Geometry: see drawing. Coordinates: mm, zero at the bounding-box minimum. A direction names the side the tool comes from. Give positions to 0.01 mm unless a question says otherwise; leave off trailing zeros. Loops run counter-clockwise (first coordinate to the right, second up) from the corner with the lowest first, then second, coordinate; pieces in that order, holes last. Notation, with made-up numbers: M 84,-10 L 139,-10 A32 cw 139,16 Z; hole C 66,-21.5 d10. An arc over 180 degrees is marked long. Answer in a Markdown table with one row per item.
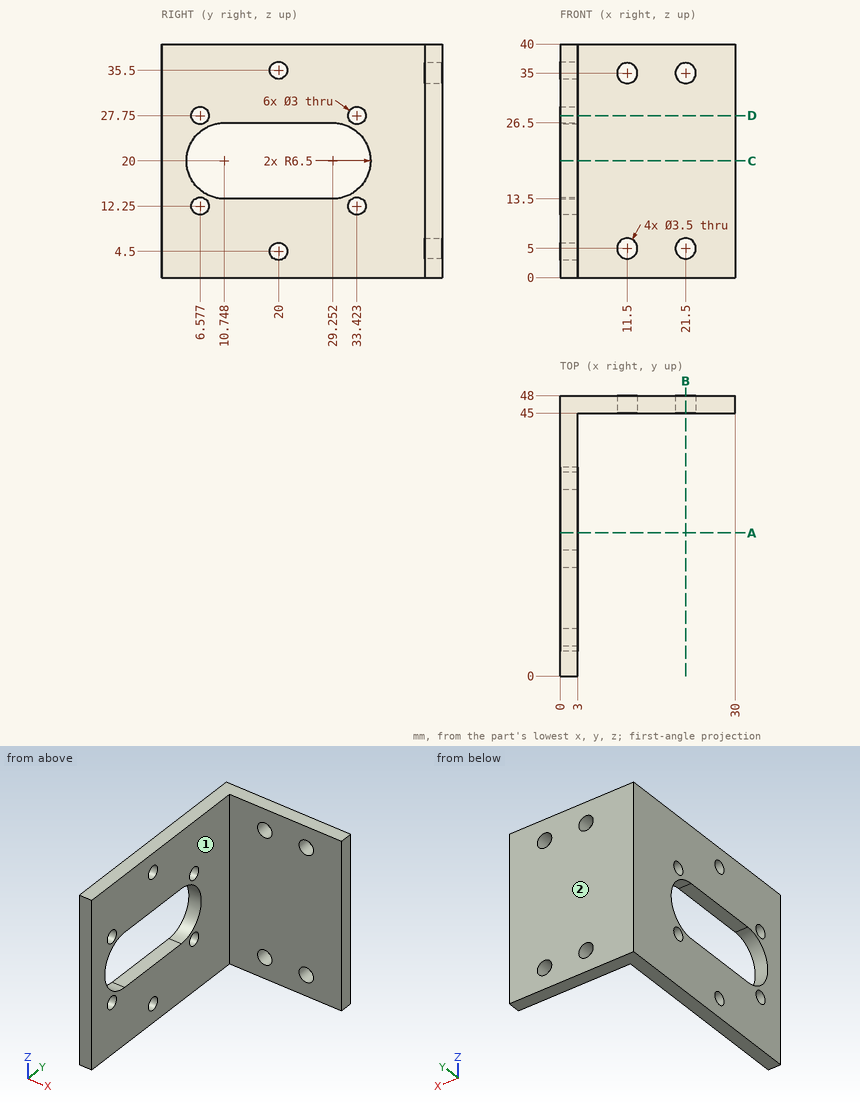
1) Section A-A, the plane y = 24.5. Return loops of the section in (x, z).
Reply:
| item | result |
|---|---|
| outline | M 0,0 L 3,0 L 3,13.5 L 0,13.5 Z; M 0,26.5 L 3,26.5 L 3,40 L 0,40 Z |
2) Section D-D, the plane z = 27.75. Return loops of the section in (x, y), then the cut area to 3 significant figures.
Reply:
| item | result |
|---|---|
| outline | M 0,0 L 3,0 L 3,5.08 L 0,5.08 Z; M 0,8.08 L 3,8.08 L 3,31.92 L 0,31.92 Z; M 0,34.92 L 3,34.92 L 3,45 L 30,45 L 30,48 L 0,48 Z |
| area | 207 mm² |
3) Material intervals for L1, parallel to X at y = 47, z = 5; L2, parallel to Z at x = 2.5, y = 14; L3, parallel to X at y = 22.5, z = 29, sorted ascending.
Reply:
| item | result |
|---|---|
| L1 | x = 0 to 9.75, 13.25 to 19.75, 23.25 to 30 |
| L2 | z = 0 to 13.5, 26.5 to 40 |
| L3 | x = 0 to 3 |
4) Section C-C, the plane z = 20. Return loops of the section in (x, y).
Reply:
| item | result |
|---|---|
| outline | M 0,0 L 3,0 L 3,4.25 L 0,4.25 Z; M 0,35.75 L 3,35.75 L 3,45 L 30,45 L 30,48 L 0,48 Z |
5) Pin query (flat end, axial travel): pin 1 Ø5.5 at (x, z) = (21.5, 35) entering from -Y; pin 2 Ø20 at (y, z) = (15.5, 27.5) entering from +X. Return the tip coordinate at first contact, or that it passes through.
Reply:
| item | result |
|---|---|
| pin 1 | stops at y = 45 |
| pin 2 | stops at x = 3 |
6) Set-up query: the marked faces 1 and 2. Return all of +Z, -Z, +X, -X, +Y, -Y with unobstructed straight access to the full face (end or side cutting, diameter ignored); none if empty.
Reply:
| item | result |
|---|---|
| face 1 | +Z, -Z, +X, -Y |
| face 2 | +Z, -Z, +X, -X, +Y |
7) Section B-B, the plane x = 21.5. Return loops of the section in (y, z).
Reply:
| item | result |
|---|---|
| outline | M 45,0 L 48,0 L 48,3.25 L 45,3.25 Z; M 45,6.75 L 48,6.75 L 48,33.25 L 45,33.25 Z; M 45,36.75 L 48,36.75 L 48,40 L 45,40 Z |
